Can you work these out from the model? Positions are in its coordinate system, mm. A direction names the side the tool comes from. Give positions to 0.01 mm unless a question says otherwise; leave off trailing zeros. Order: outer loops, then holes, each group sorted by start corner. A loop starts at its lowest first (then second) coordinate and runs counter-clockwise, first axis right, second up. Notation, with made-up numbers: M 0,61 L 31,61 A19 ccw 31,84 Z; hole C -33.5,-12 d9. An arc over 180 degrees is marked long. Write each question's results on one line, items separated by ' | '.
from build123d import *

# Parameters (mm, degrees)
SKETCH1_W           = 25.4
SKETCH1_H           = 25.4
SKETCH1_W_2         = 19.05
SKETCH1_H_2         = 19.05
EXTRUDE_THIN1_DEPTH = 660.4
SKETCH2_R           = 9.525
CUT_EXTRUDE1_DEPTH  = 662.376201568


with BuildPart() as part:
    # Sketch1 → Extrude-Thin1 (new body)
    with BuildSketch(Plane.XY):
        with Locations((-12.7, 12.7)):
            Rectangle(SKETCH1_W, SKETCH1_H)
        with Locations((-12.7, 12.7)):
            Rectangle(SKETCH1_W_2, SKETCH1_H_2, mode=Mode.SUBTRACT)
    extrude(amount=EXTRUDE_THIN1_DEPTH)

    # Sketch2 → Cut-Extrude1 (cut, through all)
    with BuildSketch(Plane.ZY.offset(25.4)):
        with Locations((25.4, 12.7)):
            Circle(SKETCH2_R)
        with Locations((177.8, 12.7)):
            Circle(SKETCH2_R)
        with Locations((482.6, 12.7)):
            Circle(SKETCH2_R)
        with Locations((635, 12.7)):
            Circle(SKETCH2_R)
        with Locations((342.9, 12.7)):
            Circle(SKETCH2_R)
    extrude(amount=-CUT_EXTRUDE1_DEPTH, mode=Mode.SUBTRACT)


solid = part.part
(1) Imagine slicing it at C-C, the plane y = 12.7. Count the separate pieces of the cut face and the enclosed holes in it, plus the area to 3 significant figures.
Data:
separate pieces: 12 | enclosed holes: 0 | area: 3,590 mm2
(2) Imagine slicing it at B-B, the plane z = 394. Write out the boundary of the cut face in (x, y) (3 decimals), plus the area to 3 significant figures.
Data:
outline: M -25.4,0 L 0,0 L 0,25.4 L -25.4,25.4 Z; hole M -22.225,3.175 L -3.175,3.175 L -3.175,22.225 L -22.225,22.225 Z | area: 282 mm2
(3) Will this pin go through, and if not, where does the flat tip stop? P1, Ø2, axis at x = -20.5, y = 18, coming from the +Z side.
Data:
P1: passes through
(4) Imagine slicing it at A-A, the plane x = -11.75. Write out the boundary of the cut face in (y, z) (3 decimals).
Data:
outline: M 0,0 L 3.175,0 L 3.175,660.4 L 0,660.4 Z; M 22.225,0 L 25.4,0 L 25.4,660.4 L 22.225,660.4 Z
(5) For faces 3 (the face through (-22.225, 13, 101)), 4 (the face through (-1.61, 9.05, 186.6)), which set-ups out of +Z, -Z, +X, -X, +Y, -Y let a thin tool reach every point of the face, with its end or its side?
Data:
face 3: +Z, -Z | face 4: +X, -X
(6) We'd pull the mould along X, two halves only. Please class faces 1 (the face through (-3.175, 13, 10)), 2 (the face through (-2, 13, 0)): +X half, -X half, draft (parallel to the pull), parting line (faces both ways), or undercut.
Data:
face 1: undercut | face 2: draft
(7) I need wall thicknesses on L1, parallel to Z at x = -23.1, y = 12.7 (3 decimals); L2, parallel to Y at x = -8.25, z = 96.5 (3 decimals); L3, parallel to X at y = 14.5, z = 86 (3 decimals). Which ranges of each line are inside material? Lowest first, please. Write a range as from..to.
Data:
L1: z = 0..15.875, 34.925..168.275, 187.325..333.375, 352.425..473.075, 492.125..625.475, 644.525..660.4 | L2: y = 0..3.175, 22.225..25.4 | L3: x = -25.4..-22.225, -3.175..0
